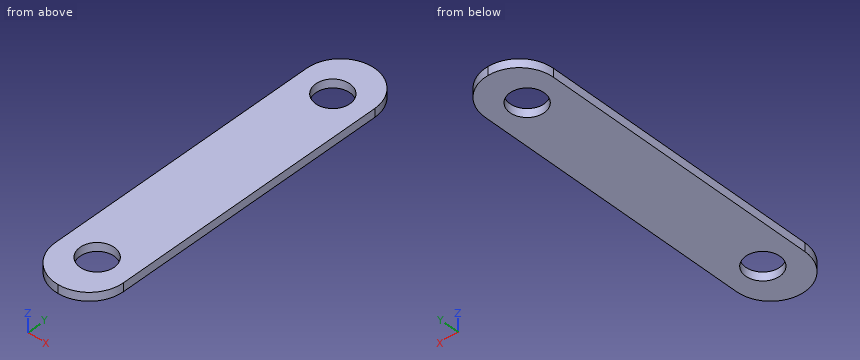
```python
from build123d import *

# Parameters (mm, degrees)
SKETCH1_W           = 4
SKETCH1_H           = 20
SKETCH1_R           = 1
BOSS_EXTRUDE1_DEPTH = 0.5
FILLET1_R           = 2
FILLET2_R           = 2
FILLET3_R           = 2
FILLET4_R           = 2


with BuildPart() as part:
    # Sketch1 → Boss-Extrude1 (new body)
    with BuildSketch(Plane.XY):
        with Locations((2, 10)):
            Rectangle(SKETCH1_W, SKETCH1_H)
        with Locations((2, 17.5)):
            Circle(SKETCH1_R, mode=Mode.SUBTRACT)
        with Locations((2, 2.5)):
            Circle(SKETCH1_R, mode=Mode.SUBTRACT)
    extrude(amount=BOSS_EXTRUDE1_DEPTH)

    # Fillet1
    fillet1_edges = [part.edges().sort_by_distance(p)[0] for p in [
        (4, 0, 0.25),
    ]]
    fillet(fillet1_edges, radius=FILLET1_R)

    # Fillet2
    fillet2_edges = [part.edges().sort_by_distance(p)[0] for p in [
        (0, 0, 0.25),
    ]]
    fillet(fillet2_edges, radius=FILLET2_R - 0.0001)  # a hair under: the kernel refuses the full size

    # Fillet3
    fillet3_edges = [part.edges().sort_by_distance(p)[0] for p in [
        (0, 20, 0.25),
    ]]
    fillet(fillet3_edges, radius=FILLET3_R)

    # Fillet4
    fillet4_edges = [part.edges().sort_by_distance(p)[0] for p in [
        (4, 20, 0.25),
    ]]
    fillet(fillet4_edges, radius=FILLET4_R - 0.0001)  # a hair under: the kernel refuses the full size


solid = part.part
```
For this review, take the finished solid that the model builds, in its own axes (mm). Coordinates: 2 decimals unless noted, no trailing zeros. Write each loop counter-clockwise with the first axis right and the second up, starting at its lowest first coordinate (ties: lowest second). Pieces come first, ordered by that corner, then holes.
(1) Add section B-B on z = 0.1. Count the separate pieces of the cut face and the enclosed holes in it, then the cut area to 3 significant figures.
(2) Add section D-D on y = 2.75. Give the boundary of the cut face in (x, z).
(3) Add section A-A on y = 17.5. Give the boundary of the cut face in (x, z).
(4) Wall thickness on probe 1 along Y at (x, z) = (1.95, 0.2); probe 2 along Y at (x, z) = (2.55, 0.35); probe 3 along Y at (x, z) = (3.6, 0.3): over which ranges is each line inside the solid? List them lowest first.
(5) Add section C-C on x = 1.4. Give the boundary of the cut face in (y, z).
Answer sheet:
1. separate pieces: 1
1. enclosed holes: 2
1. area: 70.3 mm2
2. outline: (0, 0) - (1.03, 0) - (1.03, 0.5) - (0, 0.5) - close; (2.97, 0) - (4, 0) - (4, 0.5) - (2.97, 0.5) - close
3. outline: (0, 0) - (1, 0) - (1, 0.5) - (0, 0.5) - close; (3, 0) - (4, 0) - (4, 0.5) - (3, 0.5) - close
4. probe 1: y = 0 to 1.5, 3.5 to 16.5, 18.5 to 20
4. probe 2: y = 0.08 to 1.66, 3.34 to 16.66, 18.34 to 19.92
4. probe 3: y = 0.8 to 19.2
5. outline: (0.09, 0) - (1.7, 0) - (1.7, 0.5) - (0.09, 0.5) - close; (3.3, 0) - (16.7, 0) - (16.7, 0.5) - (3.3, 0.5) - close; (18.3, 0) - (19.91, 0) - (19.91, 0.5) - (18.3, 0.5) - close
